Verification items for this drawing (mm, ordinates from the low corner). Round coordinates to 2 decimals unless told otherwise and drop trailing zeros. Loops run counter-clockwise (first coordinate to the right, second up) from the corner with the lowest first, then second, coordinate; pieces in that order, holes last. Notation, with made-up numbers: (-33, -30.5) - (26, -30.5) arc R20 ccw to (26, -8.5) - close; hole circle Ø2 at (26, 67.5). An arc over 180 degrees is marked (long way). Answer in a Markdown table with one row per item. Add a question column.
(1) Mould release check, pull along Y, two halves, no side actions. Record for the marked faces 1, 2 and 3: +Y half, -Y half, draft (parallel to the pull), parting line (faces both ways), or undercut.
(2) Gauge pin test, flat ends, axial feed: pin 1 (1.5 mm diameter, centred on x = 48.5, z = 3.5, fed in from -Y); pin 2 (3 mm diameter, centred on y = 1.5, z = 3, fed in from -X); pin 3 (3 mm diameter, centred on x = 26.5, y = 7, fed in from -Z). Record the tip position at first contact, or that the pin passes through.
(3) Cross-section at B-B on y = 5. Enter the section's corners in (x, z).
(4) Cross-section at D-D on x = 63. Enter the section's corners in (y, z).
(5) Cross-section at C-C on z = 2.5. Enter the section's corners in (x, y), then the cut area to 3 significant figures.
(6) Cross-section at A-A on x = 5. Enter the section's corners in (y, z).
(7) Thickness scan on line 1 along Y through (x, z) = (5, 2.05); line 2 along X through (y, z) = (5.25, 0.75); line 3 along X through (y, z) = (8, 3.05). Record the ranges inside material, lowest first.
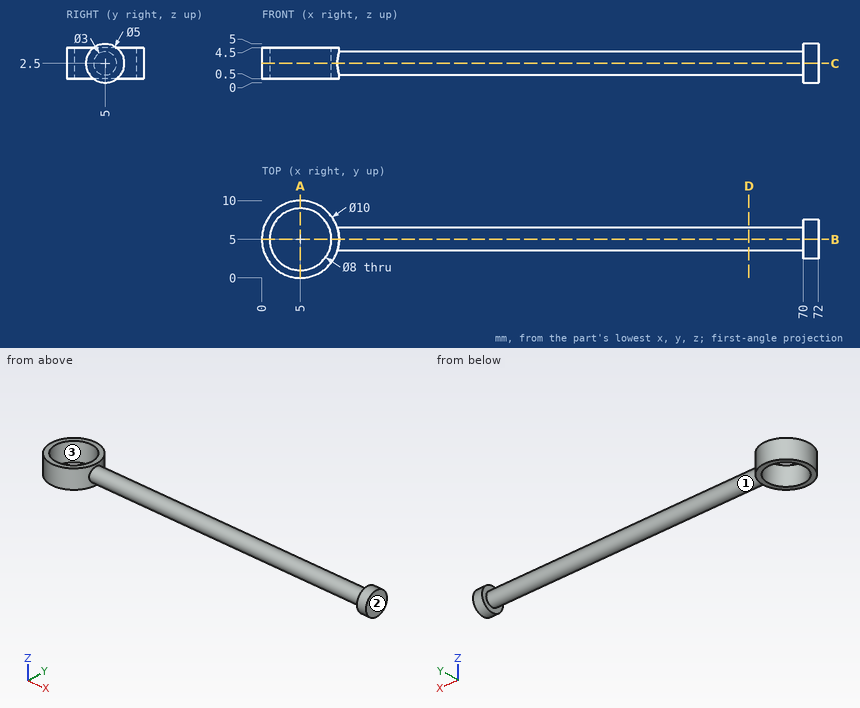
Answers:
| question | item | result |
|---|---|---|
| 1 | face 1 | parting line |
| 1 | face 2 | draft |
| 1 | face 3 | undercut |
| 2 | pin 1 | stops at y = 3.52 |
| 2 | pin 2 | stops at x = 0.42 |
| 2 | pin 3 | stops at z = 1.09 |
| 3 | outline | (0, 0.5) - (1, 0.5) - (1, 4.5) - (0, 4.5) - close; (9, 0.5) - (10, 0.5) - (10, 1) - (70, 1) - (70, 0) - (72, 0) - (72, 5) - (70, 5) - (70, 4) - (10, 4) - (10, 4.5) - (9, 4.5) - close |
| 4 | outline | circle Ø3 at (5, 2.5) |
| 5 | outline | (9.77, 3.5) - (70, 3.5) - (70, 2.5) - (72, 2.5) - (72, 7.5) - (70, 7.5) - (70, 6.5) - (9.77, 6.5) arc R5 ccw (long way) to start; hole circle Ø8 at (5, 5) |
| 5 | area | 219 mm^2 |
| 6 | outline | (0, 0.5) - (1, 0.5) - (1, 4.5) - (0, 4.5) - close; (9, 0.5) - (10, 0.5) - (10, 4.5) - (9, 4.5) - close |
| 7 | line 1 | y = 0 to 1, 9 to 10 |
| 7 | line 2 | x = 0.01 to 1.01, 8.99 to 9.99, 70 to 72 |
| 7 | line 3 | x = 1 to 2.35, 7.65 to 9 |
